from build123d import *

# Parameters (mm, degrees)
SKETCH5_W           = 100
SKETCH5_H           = 100
BOSS_EXTRUDE1_DEPTH = 5
BOSS_EXTRUDE2_DEPTH = 12


with BuildPart() as part:
    # Sketch5 → Boss-Extrude1 (new body)
    with BuildSketch(Plane(origin=(0, 0, 0), x_dir=(1, 0, 0), z_dir=(0, 1, 0))):
        with Locations((50, 50)):
            Rectangle(SKETCH5_W, SKETCH5_H)
    extrude(amount=BOSS_EXTRUDE1_DEPTH)

    # Sketch7 → Boss-Extrude2 (add)
    with BuildSketch(Plane(origin=(0, 5, 0), x_dir=(1, 0, 0), z_dir=(0, 1, 0))):
        with BuildLine():
            ThreePointArc((81.180339887, 60), (80.606601718, 80.606601718), (60, 81.180339887))
            ThreePointArc((60, 81.180339887), (50, 77.360679775), (40, 81.180339887))
            ThreePointArc((40, 81.180339887), (19.393398282, 80.606601718), (18.819660113, 60))
            ThreePointArc((18.819660113, 60), (22.639320225, 50), (18.819660113, 40))
            ThreePointArc((18.819660113, 40), (19.393398282, 19.393398282), (40, 18.819660113))
            ThreePointArc((40, 18.819660113), (50, 22.639320225), (60, 18.819660113))
            ThreePointArc((60, 18.819660113), (80.606601718, 19.393398282), (81.180339887, 40))
            ThreePointArc((81.180339887, 40), (77.360679775, 50), (81.180339887, 60))
        make_face()
    extrude(amount=BOSS_EXTRUDE2_DEPTH)


solid = part.part
Input: part model. Units: mm. Frame: model coordinates. A direction names the side the tool comes from. Coordinates: 2 decimals unless noted, no trailing zeros. Loops run counter-clockwise (first coordinate to the right, second up) from the corner with the lowest first, then second, coordinate; pieces in that order, holes last. Notation, with made-up numbers: (-6.75, -10) -> (33.25, -10) arc R10 ccw to (33.25, 5) -> close; hole circle Ø7 at (77.25, 5.25). An arc over 180 degrees is marked (long way). Write item = value, one per line. Start each with the question number.
Item 1: Cut plane B-B, the plane z = -30. Return loops of the section in (x, y), plus the area to 3 significant figures.
Item 2: First-contact query: P1, Ø3, axis at x = 47, z = -82.5, coming from the +Y side; P2, Ø1.5, axis at y = 6.5, z = -30.5, coming from the -X side; P3, Ø4, axis at x = 17, y = 8, coming from the +Z side; P4, Ø8, axis at x = 11.5, z = -29, coming from the +Y side. Flat tips, straight axial feed; report the tip coordinate or a pass-through.
Item 3: Cut plane D-D, the plane x = 89. Return loops of the section in (y, z), plus the area to 3 significant figures.
Item 4: Cut plane C-C, the plane z = -88. Return loops of the section in (x, y), plus the area to 3 significant figures.
Item 5: Reachability of faces 1 (the face through (0, 2, -49)), 2 (the face through (83, 5, -51)) from +Z, -Z, +X, -X, +Y, -Y: full face, straight path, thin tool, end or side. Return the list, or none.
Item 6: Cut plane A-A, the plane x = 70. Return loops of the section in (y, z), plus the area to 3 significant figures.
Item 7: Material intervals for line 1 (Y direction, x = 34, z = -9); line 2 (X direction, y = 6.75, z = -81.5); line 3 (Z direction, x = 82, y = 11), sorted ascending.
Ans:
q1.outline = (0, 0) -> (100, 0) -> (100, 5) -> (85, 5) -> (85, 17) -> (15, 17) -> (15, 5) -> (0, 5) -> close
q1.area = 1,340 mm²
q2.P1 = 5
q2.P2 = 15
q2.P3 = -19.8
q2.P4 = 17
q3.outline = (0, -100) -> (5, -100) -> (5, 0) -> (0, 0) -> close
q3.area = 500 mm²
q4.outline = (0, 0) -> (100, 0) -> (100, 5) -> (0, 5) -> close
q4.area = 500 mm²
q5.face_1 = +Z, -Z, -X, +Y, -Y
q5.face_2 = +Y
q6.outline = (0, -100) -> (5, -100) -> (5, -85) -> (17, -85) -> (17, -15) -> (5, -15) -> (5, 0) -> (0, 0) -> close
q6.area = 1,340 mm²
q7.line_1 = 0 to 5
q7.line_2 = 20.37 to 39.63, 60.37 to 79.63
q7.line_3 = -79 to -61, -39 to -21
